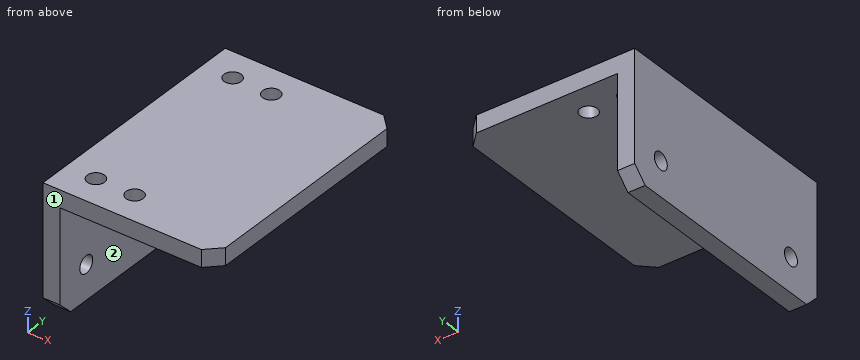
```python
from build123d import *

# Parameters (mm, degrees)
F1_DEPTH = 88.9
F3_D     = 6.35
F4_SIZE  = 5.08
F6_D     = 6.35


with BuildPart() as f1:
    # F0 (on Front) → F1 (new body)
    with BuildSketch(Plane.XZ):
        Polygon((0, 45.871365), (0, 0), (6.35, 0), (6.35, 39.521365), (63.5, 39.521365), (63.5, 45.871365), align=None)
    extrude(amount=F1_DEPTH)

    # F3 (through all)
    with Locations(Plane.YZ.offset(6.35)):
        with Locations((-76.2, 12.7), (-12.7, 12.7)):
            Hole(F3_D / 2)

    # F4
    f4_edges = [f1.edges().sort_by_distance(p)[0] for p in [
        (3.175, 0, 0),
        (3.175, -88.9, 0),
        (63.5, -88.9, 42.696365),
        (63.5, 0, 42.696365),
    ]]
    chamfer(f4_edges, length=F4_SIZE)

    # F6 (through all)
    with Locations(Plane.XY.offset(45.871365)):
        with Locations((11.1252, -11.1252), (25.4, -11.1252), (25.4, -77.8002), (11.1252, -77.8002)):
            Hole(F6_D / 2)


solid = f1.part
```
Geometry: final body of the model. Coordinates: model frame, mm. Face numbers are marked on the shaded views. A direction names the side the tool comes from. Coordinates: 2 decimals unless noted, no trailing zeros. Order: outer loops, then holes, each group sorted by start corner. A loop starts at its lowest first (then second) coordinate and runs counter-clockwise, first axis right, second up. Notation, with made-up numbers: M -22,-4.75 L 10,-4.75 A19 cw 10,-0.75 Z; hole C 31.25,-18.5 d9. An arc over 180 degrees is marked long. Answer in a Markdown table with one row per item. Add a question column.
Q1. Section query B-B on x = 25.4. Return the cut outline in (y, z), and give its area (3 significant figures).
Q2. Section query C-C on y = -76.2. Return the cut outline in (x, z) (3 decimals).
Q3. Contact query for flat-ended pins moving along their axis: P1, Ø6, axis at y = -46.5, z = 11.5, coming from the -X side; P2, Ø5.5, axis at x = 25.4, y = -77.8, coming from the +Z side; P3, Ø3, axis at x = 22.5, y = -78, coming from the -Z side; P4, Ø1, axis at y = -20.5, z = 11, coming from the +X side. Output: stop coordinate, or through.
Q4. Section query D-D on y = -33. Return the cut outline in (x, z).
Q5. Reachability of the marked faces 1 and 2 from +Z, -Z, +X, -X, +Y, -Y: full face, straight path, thin tool, end or side. Return the list, or none.
Q6. Section query A-A on z = 12.7. Return the cut outline in (x, y) (3 decimals).
Q7. Line query: L1, parallel to Y at x = 25.4, z = 43.25; L2, parallel to Z at x = 4.5, y = -12.7 (3 decimals); L3, parallel to Y at x = 3, z = 12. Output: solid intervals per line, ascending.
Completed:
| question | item | result |
|---|---|---|
| 1 | outline | M -88.9,39.52 L -80.98,39.52 L -80.98,45.87 L -88.9,45.87 Z; M -74.63,39.52 L -14.3,39.52 L -14.3,45.87 L -74.63,45.87 Z; M -7.95,39.52 L 0,39.52 L 0,45.87 L -7.95,45.87 Z |
| 1 | area | 484 mm2 |
| 2 | outline | M 0,0 L 6.35,0 L 6.35,9.525 L 0,9.525 Z; M 0,15.875 L 6.35,15.875 L 6.35,39.521 L 8.383,39.521 L 8.383,45.871 L 0,45.871 Z; M 13.867,39.521 L 22.658,39.521 L 22.658,45.871 L 13.867,45.871 Z; M 28.142,39.521 L 63.5,39.521 L 63.5,45.871 L 28.142,45.871 Z |
| 3 | P1 | stops at x = 0 |
| 3 | P2 | passes through |
| 3 | P3 | stops at z = 39.52 |
| 3 | P4 | stops at x = 6.35 |
| 4 | outline | M 0,0 L 6.35,0 L 6.35,39.52 L 63.5,39.52 L 63.5,45.87 L 0,45.87 Z |
| 5 | face 1 | +Z, -Z, +X, -X, -Y |
| 5 | face 2 | -Z, +X, +Y, -Y |
| 6 | outline | M 0,-88.9 L 6.35,-88.9 L 6.35,-79.375 L 0,-79.375 Z; M 0,-73.025 L 6.35,-73.025 L 6.35,-15.875 L 0,-15.875 Z; M 0,-9.525 L 6.35,-9.525 L 6.35,0 L 0,0 Z |
| 7 | L1 | y = -88.9 to -80.98, -74.63 to -14.3, -7.95 to 0 |
| 7 | L2 | z = 0 to 9.525, 15.875 to 45.871 |
| 7 | L3 | y = -88.9 to -79.3, -73.1 to -15.8, -9.6 to 0 |
